```python
from build123d import *

# Parameters (mm, degrees)
F0_W     = 80
F0_H     = 50
F1_DEPTH = 50
F3_DEPTH = 10
F5_DEPTH = 10
F7_DEPTH = 25
F9_DEPTH = 25


with BuildPart() as f1:
    # F0 (on Front) → F1 (new body)
    with BuildSketch(Plane.XZ):
        with Locations((-40, 25)):
            Rectangle(F0_W, F0_H)
    extrude(amount=F1_DEPTH)

    # F2 (on face) → F3 (cut)
    with BuildSketch(Plane(origin=(0, 0, 0), x_dir=(1, 0, 0), z_dir=(0, 0, -1))):
        Polygon((-30, 50), (-60, 50), (-50, 0), (-40, 0), align=None)
    extrude(amount=-F3_DEPTH, mode=Mode.SUBTRACT)

    # F4 (on face) → F5 (cut)
    with BuildSketch(Plane.XY.offset(50)):
        Polygon((-40, 0), (-30, -50), (-20, -50), (-10, 0), align=None)
    extrude(amount=-F5_DEPTH, mode=Mode.SUBTRACT)

    # F6 (on face) → F7 (cut)
    with BuildSketch(Plane.YZ):
        Polygon((-29, 35), (-44, 35), (-44, 25), (-24, 25), align=None)
    extrude(amount=-F7_DEPTH, mode=Mode.SUBTRACT)

    # F8 (on face) → F9 (cut)
    with BuildSketch(Plane.YZ):
        Polygon((0, 10), (-12, 0), (0, 0), align=None)
    extrude(amount=-F9_DEPTH, mode=Mode.SUBTRACT)

    # F13: sweep along a path in F12
    with BuildLine(Plane.XY.offset(50)) as f13_path:
        Line((-60, 0), (-50, -50))
    # F10 (on face) → F13 (sweep, cut)
    with BuildSketch(Plane.XZ.offset(50)):
        Polygon((-50, 50), (-80, 50), (-80, 15), align=None)
    sweep(path=f13_path.line, mode=Mode.SUBTRACT)


solid = f1.part
```
The listing builds one solid part. Answer for the finished solid, in the listing's coordinates (mm). A direction names the side the tool comes from. Give positions to 0.01 mm unless a question says otherwise; leave off trailing zeros. Order: outer loops, then holes, each group sorted by start corner. A loop starts at its lowest first (then second) coordinate and runs counter-clockwise, first axis right, second up. Notation, with made-up numbers: (12, 2) -> (24, 2) arc R36 ccw to (24, 37) -> close; hole circle Ø10 at (43.25, 10.5). An arc over 180 degrees is marked (long way). Answer as a JSON object with one key per item and string values. Group by question number.
Item 1: The part is cut by section A-A on x = -17. Write down the section's boundary in (y, z), and give its area (4 significant figures).
Item 2: Determine the mould class of faces 4 (the flat face through (-25, -19, 40)), 5 (the flat face through (-15, -25, 45)), 6 (the flat face through (-12.325, -26.465, 29.93)) for opening direction Y: pulls with the +Y half, pulls with the -Y half, needs draft (parallel to the pull), parting line crosses it, or undercut.
Item 3: The part is cut by section C-C on z = 34. Write down the section's boundary in (x, y).
Item 4: A tool of negligible diameter and unlimited length cuts with its end or side. For faces 1 (the flat face through (-45, -31, 10)), 2 (the flat face through (-12, -36, 35)), 3 (the flat face through (-12, -6, 5)), from which of +Z, -Z, +X, -X, +Y, -Y can it reach the whole face along a straight path? Write none if from no direction.
Item 5: Flat-ended cylindrical pins translate along their axes: pin 1 (1.5 mm diameter, centred on x = -20.5, y = -26, fed in from -Z); pin 2 (3 mm diameter, centred on y = -34.5, z = 29, fed in from +X). Find the tip coordinate at first contact, or state that the pin passes through.
Item 6: Consider L1, parallel to Z at x = -19, y = -38; L2, parallel to Z at x = -35, y = -3; L3, parallel to Z at x = -50, y = -4. Determine where each line is inside the solid, lowest interval first. Write a range as from..to.
Item 7: The part is cut by section D-D on y = -4. Write down the section's boundary in (x, z).
Item 8: The part is cut by section B-B on z = 42.5. Write down the section's boundary in (x, y).
Result set:
{
 "1": {"outline": "(-50, 0) -> (-12, 0) -> (0, 10) -> (0, 40) -> (-35, 40) -> (-35, 50) -> (-50, 50) -> close; hole (-44, 25) -> (-24, 25) -> (-29, 35) -> (-44, 35) -> close", "area": "1,915 mm²"},
 "2": {"face 4": "needs draft", "face 5": "pulls with the +Y half", "face 6": "undercut"},
 "3": {"outline": "(-73.71, 0) -> (-63.71, -50) -> (0, -50) -> (0, -44) -> (-25, -44) -> (-25, -28.5) -> (0, -28.5) -> (0, 0) -> close"},
 "4": {"face 1": "-Z, -Y", "face 2": "+X", "face 3": "-Z, +X, +Y"},
 "5": {"pin 1": "z = 0", "pin 2": "x = -25"},
 "6": {"L1": "0..25, 35..40", "L2": "0..40", "L3": "10..50"},
 "7": {"outline": "(-80, 0) -> (-50.8, 0) -> (-50.8, 10) -> (-39.2, 10) -> (-39.2, 0) -> (-25, 0) -> (-25, 6.67) -> (0, 6.67) -> (0, 50) -> (-10.8, 50) -> (-10.8, 40) -> (-39.2, 40) -> (-39.2, 50) -> (-59.2, 50) -> (-80, 25.73) -> close"},
 "8": {"outline": "(-66.43, 0) -> (-56.43, -50) -> (-30, -50) -> (-40, 0) -> close; (-20, -50) -> (0, -50) -> (0, 0) -> (-10, 0) -> close"}
}
